Check sheet for the modelled part. Datum: model origin and axes. Units: mm. A direction names the side the tool comes from. Round coordinates to 2 decimals unless told otherwise and drop trailing zeros. Order: outer loops, then holes, each group sorted by start corner. A loop starts at its lowest first (then second) coordinate and runs counter-clockwise, first axis right, second up.
```python
from build123d import *

# Parameters (mm, degrees)
SKIZZE2_OUTSIDE_W               = 26.122
SKIZZE2_OUTSIDE_H               = 26.122
SCHNITT_LINEAR_AUSTRAGEN1_DEPTH = 42.674393343


with BuildPart() as part:
    # Skizze1 → Basis-Rotation (revolve)
    with BuildSketch(Plane.XY, mode=Mode.PRIVATE) as basis_rotation_sk:
        Polygon((0, 5.3), (0, -35), (3.3865, -35), (3.3865, -3), (3.998, -0.002), (4, -0.002), (4, 0), (6.5, 0), (6.5, 0.6), (7.5055, 0.6), (7.5055, 4.719474304), (6.5, 5.3), align=None)
    revolve(basis_rotation_sk.sketch.rotate(Axis((0, 5.3, 0), (0, -1, 0)), 180), axis=Axis((0, 5.3, 0), (0, -1, 0)))

    # Skizze2 outside → Schnitt-Linear austragen1 (cut, through all)
    with BuildSketch(Plane(origin=(0, 5.3, 0), x_dir=(-1, 0, 0), z_dir=(0, 1, 0))):
        Rectangle(SKIZZE2_OUTSIDE_W, SKIZZE2_OUTSIDE_H)
        Polygon((-3.75277675, 6.5), (3.75277675, 6.5), (7.505553499, 0), (3.75277675, -6.5), (-3.75277675, -6.5), (-7.505553499, 0), align=None, mode=Mode.SUBTRACT)
    extrude(amount=-SCHNITT_LINEAR_AUSTRAGEN1_DEPTH, mode=Mode.SUBTRACT)


solid = part.part
```
Item 1: Go/stop test with flat-tipped pins: P1, Ø1.5, axis at x = -6.5, z = 0, coming from the -Y side; P2, Ø1.5, axis at y = 1, z = -4.5, coming from the +X side; P3, Ø6, axis at y = -17, z = 1.5, coming from the +X side; P4, Ø4, axis at x = -2, z = -3, coming from the -Y side. Record where each tip stops, or that it passes through.
Answer:
P1: stops at y = 0
P2: stops at x = 5.34
P3: stops at x = 3.39
P4: stops at y = -35
Item 2: Scan lines: line 1 along Y through (x, z) = (-2.25, -5); line 2 along Z through (x, y) = (0.25, -17). Record each from-to range of solid material in increasing order.
Answer:
line 1: y = 0 to 5.3
line 2: z = -3.38 to 3.38
Item 3: Sectioned sample at A-A (y = -11.5). Record the cut outline in (x, z), and give its area (3 significant figures).
Answer:
outline: circle Ø6.77 at (0, 0)
area: 36.0 mm2
Item 4: Access from +Z, -Z, +X, -X, +Y, -Y to the whole of each face (thin tool, end or side, straight path). Record for faces 1 (the flat face through (-3, 0.6, -6)), 2 (the conical face through (3.38, 5.16, 5.83)), 3 (the flat face through (3, 0.6, 6)), 4 (the flat face through (7, 0.6, 0)), 5 (the cylindrical face through (2.496, -18.776, -2.289)).
Answer:
face 1: -Z, -X, -Y
face 2: +Z, +X, +Y
face 3: +Z, +X, -Y
face 4: +X, -Y
face 5: -Y
